Geometry check sheet. Reference: drawing and pictorial views, mm from the part's lowest x, y, z. A direction names the side the tool comes from. Round coordinates to 2 decimals unless told otherwise and drop trailing zeros. Order: outer loops, then holes, each group sorted by start corner. A loop starts at its lowest first (then second) coordinate and runs counter-clockwise, first axis right, second up.
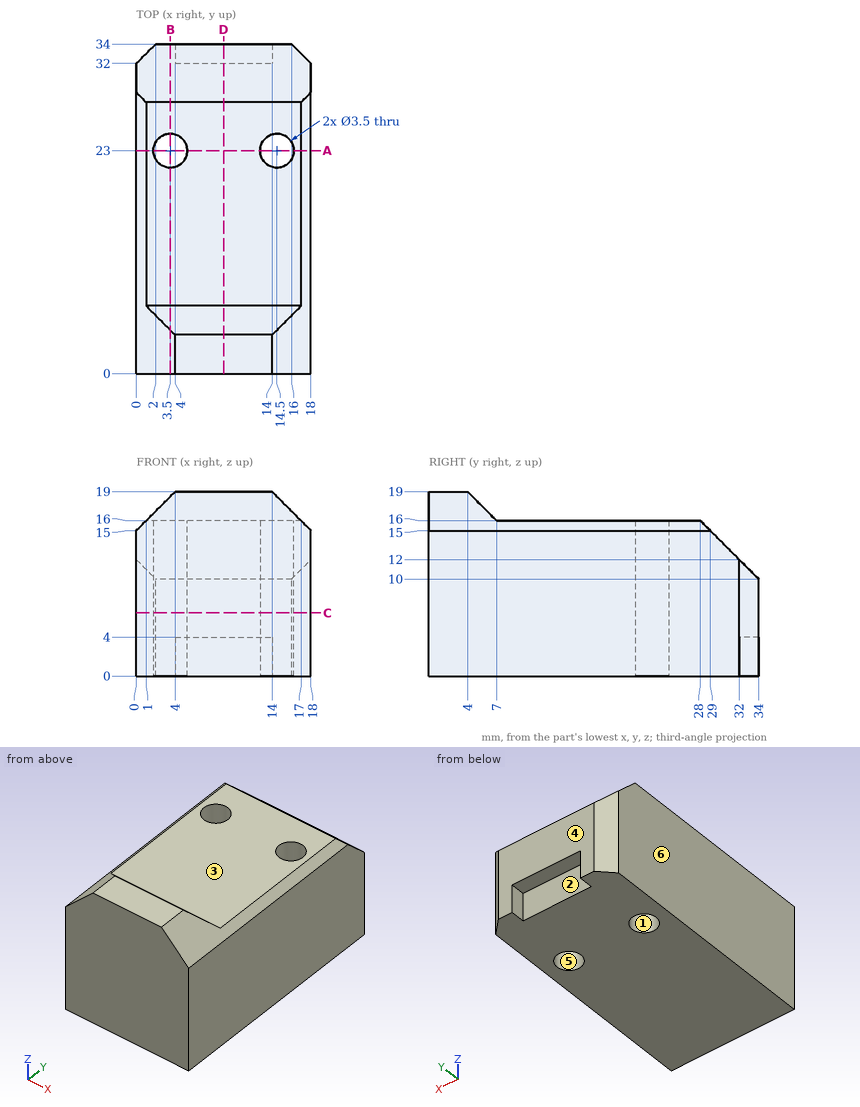
1) Go/stop test with flat-tipped pins: pin 1 Ø5.5 at (x, y) = (3.5, 23) entering from +Z; pin 2 Ø1.6 at (x, y) = (10, 33) entering from -Z; pin 3 Ø1.5 at (x, z) = (8, 16) entering from +Y. Record where each tip stops, or that it passes through.
2) Sectioned sample at C-C on z = 6.5. Record the cut outline in (x, y), then the cut area to 3 significant figures.
3) Draft check along Y on the marked faces 4, 5 and 6. Enter one of: released by +Y, released by -Y, zero draft, split by the parting line, or undercut.
4) Sectioned sample at D-D on x = 9. Record the cut outline in (y, z), then the cut area to 4 significant figures.
5) Sectioned sample at A-A on y = 23. Record the cut outline in (x, z).
6) Scan lines: probe 1 along X at (y, z) = (23, 11.25); probe 2 along Y at (x, z) = (3.5, 8.5); probe 3 along Z at (x, y) = (4, 28). Record each from-to range of solid material in increasing order.
7) Tool access check on the marked faces 1, 2 and 3. Record the directions out of +Z, -Z, +X, -X, +Y, -Y that give a thin tool (end or side, any length) a straight path to the whole face; none if there is none.
8) Sectioned sample at B-B on x = 3.5. Record the cut outline in (y, z).
Returned:
1. pin 1: stops at z = 16
1. pin 2: stops at z = 4
1. pin 3: stops at y = 28.75
2. outline: (0, 0) - (18, 0) - (18, 32) - (16, 34) - (2, 34) - (0, 32) - close; hole circle Ø3.5 at (3.5, 23); hole circle Ø3.5 at (14.5, 23)
2. area: 589 mm2
3. face 4: released by +Y
3. face 5: undercut
3. face 6: zero draft
4. outline: (0, 0) - (32, 0) - (32, 4) - (34, 4) - (34, 10) - (28, 16) - (7, 16) - (4, 19) - (0, 19) - close
4. area: 534.5 mm2
5. outline: (0, 0) - (1.75, 0) - (1.75, 16) - (1, 16) - (0, 15) - close; (5.25, 0) - (12.75, 0) - (12.75, 16) - (5.25, 16) - close; (16.25, 0) - (18, 0) - (18, 15) - (17, 16) - (16.25, 16) - close
6. probe 1: x = 0 to 1.75, 5.25 to 12.75, 16.25 to 18
6. probe 2: y = 0 to 21.25, 24.75 to 34
6. probe 3: z = 0 to 16
7. face 1: +Z, -Z
7. face 2: -Z, +Y
7. face 3: +Z, +X, -X, +Y
8. outline: (0, 0) - (21.25, 0) - (21.25, 16) - (7, 16) - (4.5, 18.5) - (0, 18.5) - close; (24.75, 0) - (34, 0) - (34, 10) - (28, 16) - (24.75, 16) - close
